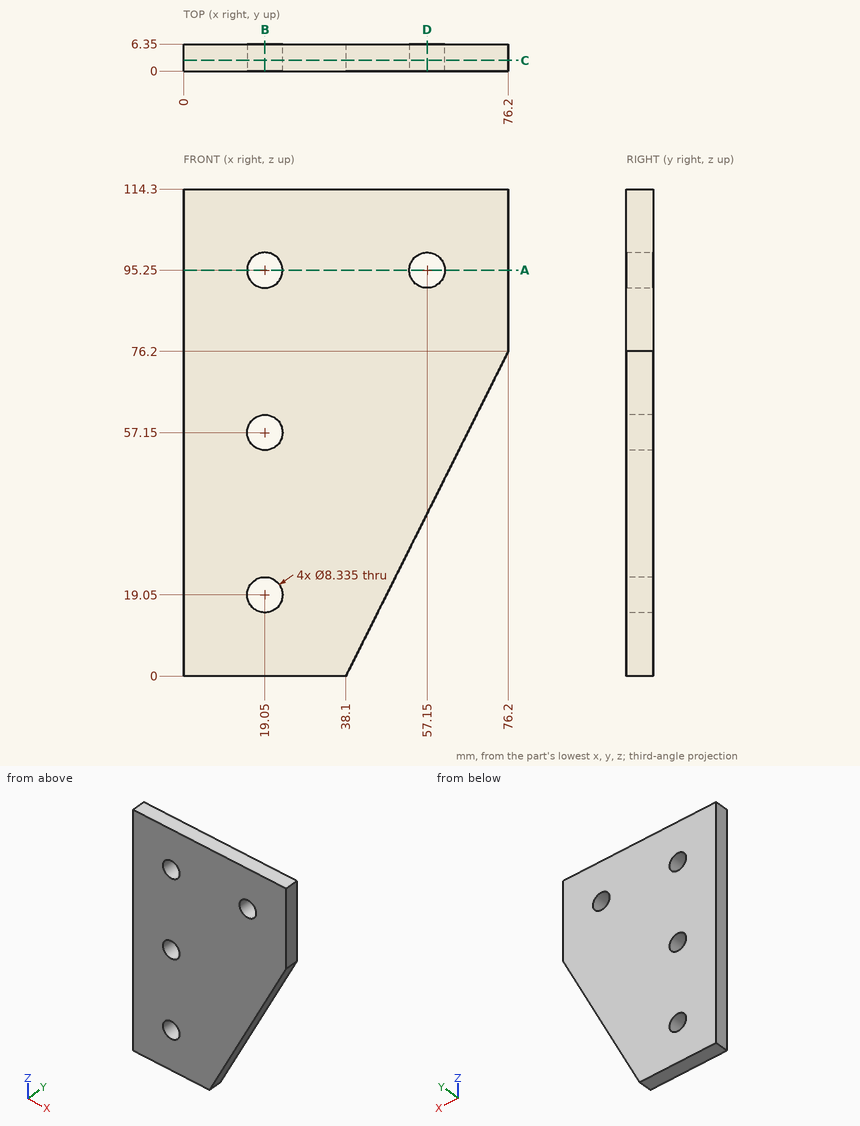
Geometry: see drawing. Coordinates: mm, zero at the bounding-box minimum. Give positions to 0.01 mm unless a question says otherwise; leave off trailing zeros. Write each loop counter-clockwise with the first axis right and the second up, starting at its lowest first coordinate (ties: lowest second). Pieces come first, ordered by that corner, then holes. Notation, with made-up numbers: M 89.25,18 L 93.25,18 A19 ccw 93.25,23 Z; hole C -10,80 d6. An arc over 180 degrees is marked long. Answer in a Markdown table with one row per item. Add a question column.
(1) First-contact query: pin 1 (1.5 mm diameter, centred on y = 3.5, z = 68.5, fed in from +X) (1 decimal). Flat tip, straight axial feed; report the tip coordinate or a pass-through.
(2) Section B-B on x = 19.05. Return loops of the section in (y, z), and give its area (3 significant figures).
(3) Section D-D on x = 57.15. Return loops of the section in (y, z).
(4) Section A-A on z = 95.25. Return loops of the section in (x, y), and give its area (3 significant figures).
(5) Section C-C on y = 2.5. State how many separate pieces and enclosed holes the cut face has, and give its area (3 significant figures).
(6) Ray query, line 1 (Z direction, x = 19.05, y = 2); line 2 (X direction, y = 1.75, z = 95.25); line 3 (Z direction, x = 57.15, y = 3.25) (1 decimal). Return the intervals inside material, ascending.
Result set:
| question | item | result |
|---|---|---|
| 1 | pin 1 | stops at x = 72.7 |
| 2 | outline | M 0,0 L 6.35,0 L 6.35,14.88 L 0,14.88 Z; M 0,23.22 L 6.35,23.22 L 6.35,52.98 L 0,52.98 Z; M 0,61.32 L 6.35,61.32 L 6.35,91.08 L 0,91.08 Z; M 0,99.42 L 6.35,99.42 L 6.35,114.3 L 0,114.3 Z |
| 2 | area | 567 mm^2 |
| 3 | outline | M 0,38.1 L 6.35,38.1 L 6.35,91.08 L 0,91.08 Z; M 0,99.42 L 6.35,99.42 L 6.35,114.3 L 0,114.3 Z |
| 4 | outline | M 0,0 L 14.88,0 L 14.88,6.35 L 0,6.35 Z; M 23.22,0 L 52.98,0 L 52.98,6.35 L 23.22,6.35 Z; M 61.32,0 L 76.2,0 L 76.2,6.35 L 61.32,6.35 Z |
| 4 | area | 378 mm^2 |
| 5 | separate pieces | 1 |
| 5 | enclosed holes | 4 |
| 5 | area | 7,040 mm^2 |
| 6 | line 1 | z = 0 to 14.88, 23.22 to 52.98, 61.32 to 91.08, 99.42 to 114.3 |
| 6 | line 2 | x = 0 to 14.88, 23.22 to 52.98, 61.32 to 76.2 |
| 6 | line 3 | z = 38.1 to 91.1, 99.4 to 114.3 |
